Autodesk Inventor part; units mm, degrees
ref_plane "YZ Plane" through (0, 0, 0) normal (1, 0, 0) x (0, 1, 0)
ref_plane "XZ Plane" through (0, 0, 0) normal (0, 1, 0) x (-1, 0, 0)
ref_plane "XY Plane" through (0, 0, 0) normal (0, 0, 1) x (1, 0, 0)
sketch "Sketch1" plane through (0, 0, 0) normal (0, 1, 0) x (-1, 0, 0)
  line L0 (0, -19.05) -> (0, -158.75)
  line L1 (19.05, -177.8) -> (19.05, -177.8)
  line L2 (38.1, -158.75) -> (38.1, -19.05)
  line L3 (19.05, 0) -> (19.05, 0)
  arc A0 (0, -158.75) -> (19.05, -177.8) centre (19.05, -158.75) ccw
  arc A1 (19.05, -177.8) -> (38.1, -158.75) centre (19.05, -158.75) ccw
  arc A2 (38.1, -19.05) -> (19.05, 0) centre (19.05, -19.05) ccw
  arc A3 (19.05, 0) -> (0, -19.05) centre (19.05, -19.05) ccw
  circle A4 centre (19.05, -19.05) radius 3.9688
  circle A5 centre (19.05, -158.75) radius 3.9688
  point P0 (0, 0)
  point P1 (0, -177.8)
  point P2 (38.1, -177.8)
  dimension "d0" = 38.1
  dimension "LengthOfArm_Thicker" = 177.8
  dimension "d2" = 19.05
  dimension "d3" = 7.9375
  dimension "Motor_Shaft_Diameter" = 7.9375
extrude "Extrusion1" add sketch "Sketch1" along normal blind 31.75
sketch "Sketch3" plane through (0, 0, -19.05) normal (1, 0, 0) x (0, 0, -1)
  line L0 (-57.15, 11.43) -> (19.05, 11.43)
  line L1 (19.05, 11.43) -> (19.05, 17.78)
  line L2 (19.05, 17.78) -> (-57.15, 17.78)
  line L3 (-57.15, 17.78) -> (-57.15, 11.43)
  line L4 (-19.05, 0) -> (-19.05, 31.75)
  line L5 (-57.15, 11.43) -> (19.05, 17.78) construction
  line L6 (19.05, 11.43) -> (-57.15, 17.78) construction
  line L7 (0, 0) -> (-19.05, 0)
  line L8 (-19.05, 0) -> (-19.05, 31.75)
  line L9 (-19.05, 21.59) -> (69.85, 21.59)
  line L10 (69.85, 21.59) -> (69.85, 31.75)
  line L11 (139.7, 31.75) -> (0, 31.75)
  line L12 (0, 31.75) -> (-19.05, 31.75)
  line L13 (69.85, 31.75) -> (-19.05, 31.75)
  line L14 (-19.05, 0) -> (-19.05, 31.75)
  line L15 (-19.05, 31.75) -> (-19.05, 21.59)
  point P0 (-19.05, 14.605)
  point P1 (-19.05, 14.605)
  dimension "d15" = 6.35
  dimension "d19" = 11.43
  dimension "d20" = 10.16
  dimension "d21" = 88.9
extrude "Extrusion3" cut sketch "Sketch3" against normal up to next
fillet "Fillet3" radius 12.7 1 edges at (-19.05, 21.59, -88.9)
sketch "Sketch4" plane through (0, 31.75, 0) normal (0, 1, 0) x (1, 0, 0)
  circle A0 centre (-19.05, 158.75) radius 3.9687
  line L0 (-9.6345, 157.9562) -> (-28.4655, 157.9562)
  line L1 (-28.4655, 157.9562) -> (-28.4655, 151.6062)
  line L2 (-28.4655, 151.6062) -> (-9.6345, 151.6062)
  line L3 (-9.6345, 151.6062) -> (-9.6345, 157.9562)
  line L4 (-9.6345, 157.9562) -> (-28.4655, 151.6062) construction
  line L5 (-28.4655, 157.9562) -> (-9.6345, 151.6062) construction
  point P0 (0, 0)
  point P1 (-19.05, 154.7812)
  dimension "d23" = 6.35
extrude "Extrusion4" add sketch "Sketch4" against normal up to surface (31.75 mm away) contours L0 A0 | A0 L0 L3 L2 L1 picked at (-18.2787, 156.5235)
equation "\"Thickness_Thicker\" = 2 * Thickness_Thiner"
properties part number "ArmThicker"
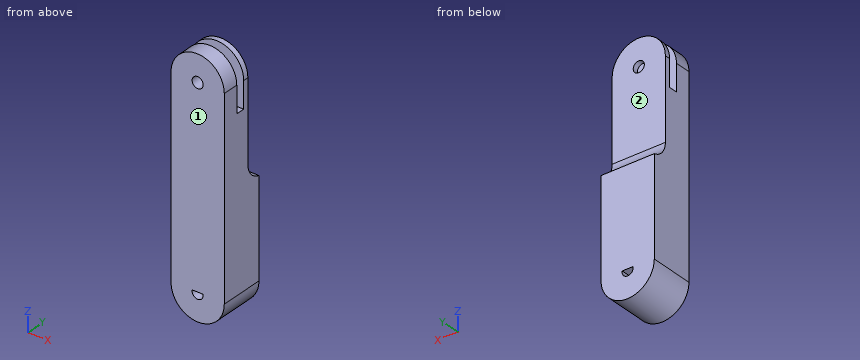
Input: part model. Units: mm. Frame: model coordinates. Face numbers are marked on the shaded views. A direction names the side the tool comes from. Give positions to 0.01 mm unless a question says otherwise; leave off trailing zeros. Write each loop counter-clockwise with the first axis right and the second up, starting at its lowest first coordinate (ties: lowest second). Pieces come first, ordered by that corner, then holes. Notation, with made-up numbers: (47.25, 12) -> (61.25, 12) arc R28 cw to (61.25, 37) -> close; hole circle Ø1 at (-25, -3). An arc over 180 degrees is marked (long way). Use one line per item in the form item = value. Start each with the question number.
1) Section query C-C on x = -7. Return the cut outline in (y, z), then the cut area to 3 significant figures.
2) Pin query (flat end, axial travel): pin 1 (11.5 mm diameter, centred on x = -22.5, z = -22, fed in from -Y); pin 2 (5 mm diameter, centred on x = -19.05, z = -19.05, fed in from -Y); pin 3 (8.5 mm diameter, centred on x = -18.5, y = 16.5, fed in from -Z); pin 4 (1 mm diameter, centred on x = -10.5, y = 24, fed in from +Z). Return the tip coordinate at first contact, or that it passes through.
3) Section query B-B on y = 15. Return the cut outline in (x, z).
4) Section query A-A on x = -19.05. Return the cut outline in (y, z), then the cut area to 3 significant figures.
5) Section query D-D on x = -28. Return the cut outline in (y, z), then the cut area to 3 significant figures.
6) Set-up query: the marked faces 1 and 2. Return all of +Z, -Z, +X, -X, +Y, -Y with unobstructed straight access to the full face (end or side cutting, diameter ignored); none if empty.
7) Ray query, probe 1 along Z at (x, y) = (-19.05, 3); probe 2 along Z at (x, y) = (-19, 13); probe 3 along Z at (x, y) = (-16, 7.5). Return the intervals inside material, ascending. Write a range as from..to.
Outcome:
q1.outline = (0, -173.5) -> (31.75, -173.5) -> (31.75, -88.9) arc R12.7 cw to (21.59, -76.46) -> (21.59, -4.3) -> (17.78, -4.3) -> (17.78, -38.1) -> (11.43, -38.1) -> (11.43, -4.3) -> (0, -4.3) -> close
q1.area = 4,330 mm^2
q2.pin_1 = 0
q2.pin_2 = through
q2.pin_3 = -177.8
q2.pin_4 = -83.15
q3.outline = (-38.1, -158.75) arc R19.05 ccw to (0, -158.75) -> (0, -38.1) -> (-38.1, -38.1) -> close; hole (-22.94, -157.96) arc R3.97 ccw (long way) to (-15.16, -157.96) -> close
q4.outline = (0, -177.8) -> (31.75, -177.8) -> (31.75, -162.72) -> (0, -162.72) -> close; (0, -157.96) -> (31.75, -157.96) -> (31.75, -88.9) arc R12.7 cw to (21.59, -76.46) -> (21.59, -23.02) -> (17.78, -23.02) -> (17.78, -38.1) -> (11.43, -38.1) -> (11.43, -23.02) -> (0, -23.02) -> close; (0, -15.08) -> (11.43, -15.08) -> (11.43, 0) -> (0, 0) -> close; (17.78, -15.08) -> (21.59, -15.08) -> (21.59, 0) -> (17.78, 0) -> close
q4.area = 4,260 mm^2
q5.outline = (0, -175.57) -> (31.75, -175.57) -> (31.75, -88.9) arc R12.7 cw to (21.59, -76.46) -> (21.59, -2.23) -> (17.78, -2.23) -> (17.78, -38.1) -> (11.43, -38.1) -> (11.43, -2.23) -> (0, -2.23) -> close
q5.area = 4,430 mm^2
q6.face_1 = +Z, -Z, +X, -X, -Y
q6.face_2 = +Z, +X, -X, +Y
q7.probe_1 = -177.8..-162.72, -157.96..-23.02, -15.08..0
q7.probe_2 = -177.8..-162.72, -157.96..-38.1
q7.probe_3 = -177.55..-161.29, -157.96..-21.59, -16.51..-0.25
